```python
from build123d import *

# Parameters (mm, degrees)
SKETCH1_W           = 25.4
SKETCH1_H           = 25.4
BOSS_EXTRUDE1_DEPTH = 5


with BuildPart() as part:
    # Sketch1 → Boss-Extrude1 (new body)
    with BuildSketch(Plane(origin=(0, 0, 0), x_dir=(1, 0, 0), z_dir=(0, 1, 0))):
        with BuildLine():
            Line((-219.790265708, 100), (-160.4, 100))
            ThreePointArc((-160.4, 100), (-146.257864376, 94.142135624), (-140.4, 80))
            Line((-140.4, 80), (-140.4, -80))
            ThreePointArc((-140.4, -80), (-146.257864376, -94.142135624), (-160.4, -100))
            Line((-160.4, -100), (-219.790265708, -100))
            ThreePointArc((-219.790265708, -100), (-217.432582206, -105.027772971), (-214.959905331, -110))
            Line((-214.959905331, -110), (-175.4, -110))
            Line((-175.4, -110), (-175.4, -115))
            Line((-175.4, -115), (-212.327014061, -115))
            ThreePointArc((-212.327014061, -115), (-170.745074453, -170.745074453), (-115, -212.327014061))
            Line((-115, -212.327014061), (-115, -175.4))
            Line((-115, -175.4), (-110, -175.4))
            Line((-110, -175.4), (-110, -214.959905331))
            ThreePointArc((-110, -214.959905331), (0, -241.47), (110, -214.959905331))
            Line((110, -214.959905331), (110, -175.4))
            Line((110, -175.4), (115, -175.4))
            Line((115, -175.4), (115, -212.327014061))
            ThreePointArc((115, -212.327014061), (170.745074453, -170.745074453), (212.327014061, -115))
            Line((212.327014061, -115), (175.4, -115))
            Line((175.4, -115), (175.4, -110))
            Line((175.4, -110), (214.959905331, -110))
            ThreePointArc((214.959905331, -110), (217.432582206, -105.027772971), (219.790265708, -100))
            Line((219.790265708, -100), (160.4, -100))
            ThreePointArc((160.4, -100), (146.257864376, -94.142135624), (140.4, -80))
            Line((140.4, -80), (140.4, 80))
            ThreePointArc((140.4, 80), (146.257864376, 94.142135624), (160.4, 100))
            Line((160.4, 100), (219.790265708, 100))
            ThreePointArc((219.790265708, 100), (217.432582206, 105.027772971), (214.959905331, 110))
            Line((214.959905331, 110), (175.4, 110))
            Line((175.4, 110), (175.4, 115))
            Line((175.4, 115), (212.327014061, 115))
            ThreePointArc((212.327014061, 115), (170.745074453, 170.745074453), (115, 212.327014061))
            Line((115, 212.327014061), (115, 175.4))
            Line((115, 175.4), (110, 175.4))
            Line((110, 175.4), (110, 214.959905331))
            ThreePointArc((110, 214.959905331), (0, 241.47), (-110, 214.959905331))
            Line((-110, 214.959905331), (-110, 175.4))
            Line((-110, 175.4), (-115, 175.4))
            Line((-115, 175.4), (-115, 212.327014061))
            ThreePointArc((-115, 212.327014061), (-170.745074453, 170.745074453), (-212.327014061, 115))
            Line((-212.327014061, 115), (-175.4, 115))
            Line((-175.4, 115), (-175.4, 110))
            Line((-175.4, 110), (-214.959905331, 110))
            ThreePointArc((-214.959905331, 110), (-217.432582206, 105.027772971), (-219.790265708, 100))
        make_face()
        with Locations((127.7, 127.7)):
            Rectangle(SKETCH1_W, SKETCH1_H, mode=Mode.SUBTRACT)
        with Locations((-127.7, 127.7)):
            Rectangle(SKETCH1_W, SKETCH1_H, mode=Mode.SUBTRACT)
        with Locations((127.7, -127.7)):
            Rectangle(SKETCH1_W, SKETCH1_H, mode=Mode.SUBTRACT)
        with Locations((-127.7, -127.7)):
            Rectangle(SKETCH1_W, SKETCH1_H, mode=Mode.SUBTRACT)
    extrude(amount=BOSS_EXTRUDE1_DEPTH)


solid = part.part
```
Source: CAD feature listing. Evaluate the final solid. Frame: model axes, mm. A direction names the side the tool comes from. Give positions to 0.01 mm unless a question says otherwise; leave off trailing zeros. Order: outer loops, then holes, each group sorted by start corner. A loop starts at its lowest first (then second) coordinate and runs counter-clockwise, first axis right, second up. Notation, with made-up numbers: (-24.75, 1) -> (-9.75, 1) arc R26 cw to (-9.75, 31) -> close; hole circle Ø3 at (47.25, -2). An arc over 180 degrees is marked (long way). Use a Markdown table: item, result.
Q1. First-contact query: P1, Ø1.5, axis at x = -134, y = 3.5, coming from the +Z side; P2, Ø3, axis at x = 97.5, y = 1, coming from the +Z side; P3, Ø10, axis at x = -123.5, z = -127.5, coming from the -Y side; P4, Ø2.5, axis at x = 133.5, y = 1.5, coming from the -Z side. Flat tips, straight axial feed; report the tip coordinate or a pass-through.
A:
| item | result |
|---|---|
| P1 | z = 201.38 |
| P2 | z = 221.57 |
| P3 | through |
| P4 | z = -202.03 |
Q2. Pull-direction query (Z, two-part tool) for faces 1 (the face through (-146.103, 2.465, 93.986)), 2 (the face through (1.599, 2.465, -241.465)), 3 (the face through (170.053, 2.465, 171.435)); classes: +Z half, -Z half, draft (parallel to the pull), parting line (faces both ways), or undercut.
A:
| item | result |
|---|---|
| face 1 | undercut |
| face 2 | -Z half |
| face 3 | +Z half |
Q3. Access query for faces 4 (the face through (146.103, 2.465, -93.986)), 5 (the face through (-1.599, 2.465, 241.465)), 6 (the face through (-146.414, 2.465, -94.297)). Directions: +Z, -Z, +X, -X, +Y, -Y. A direction counts if a zero-diameter tool reaches every point of the face in a straight line with its end or side. Return the directions, or none.
A:
| item | result |
|---|---|
| face 4 | +X, +Y, -Y |
| face 5 | +Z, +Y, -Y |
| face 6 | -X, +Y, -Y |
Q4. Section D-D (z = 205). Return the cut outline in (x, y), and give its area (3 significant figures).
A:
| item | result |
|---|---|
| outline | (-127.6, 0) -> (-115, 0) -> (-115, 5) -> (-127.6, 5) -> close; (-110, 0) -> (110, 0) -> (110, 5) -> (-110, 5) -> close; (115, 0) -> (127.6, 0) -> (127.6, 5) -> (115, 5) -> close |
| area | 1,230 mm^2 |
Q5. Section C-C (y = 3.95). State how many separate pieces and enclosed holes the cut face has, and give its area (3 significant figures).
A:
| item | result |
|---|---|
| separate pieces | 1 |
| enclosed holes | 4 |
| area | 142,000 mm^2 |
Q6. Material intervals for line 1 (Z direction, x = 140, y = 1.85); line 2 (X direction, y = 4.5, z = -132); line 3 (X direction, y = 2, z = -128), sorted ascending. Write a range as [from, to].
A:
| item | result |
|---|---|
| line 1 | [-196.74, -140.4], [-115, 115], [140.4, 196.74] |
| line 2 | [-202.2, -140.4], [-115, 115], [140.4, 202.2] |
| line 3 | [-204.75, -140.4], [-115, 115], [140.4, 204.75] |
Q7. Section B-B (z = 135). Return the cut outline in (x, y).
A:
| item | result |
|---|---|
| outline | (-200.21, 0) -> (-140.4, 0) -> (-140.4, 5) -> (-200.21, 5) -> close; (-115, 0) -> (115, 0) -> (115, 5) -> (-115, 5) -> close; (140.4, 0) -> (200.21, 0) -> (200.21, 5) -> (140.4, 5) -> close |
Q8. Section A-A (x = 148). Return the cut outline in (y, z).
A:
| item | result |
|---|---|
| outline | (0, -190.8) -> (5, -190.8) -> (5, -95.69) -> (0, -95.69) -> close; (0, 95.69) -> (5, 95.69) -> (5, 190.8) -> (0, 190.8) -> close |
